from build123d import *

# Parameters (mm, degrees)
SKETCH_W        = 100
SKETCH_H        = 84
PAD_DEPTH       = 10
SKETCH001_R     = 2.1
POCKET_DEPTH    = 10
SKETCH002_R     = 3.2
POCKET001_DEPTH = 10
SKETCH003_R     = 4
POCKET002_DEPTH = 5
POCKET003_DEPTH = 4
SKETCH004_R     = 4.9
POCKET004_DEPTH = 5.2
FILLET_R        = 2
FILLET001_R     = 0.8
FILLET002_R     = 0.8


with BuildPart() as part:
    # Sketch → Pad (new body)
    with BuildSketch(Plane.XY):
        with Locations((50, 42)):
            Rectangle(SKETCH_W, SKETCH_H)
    extrude(amount=PAD_DEPTH)

    # Sketch001 (on Face6 of Pad) → Pocket (cut)
    with BuildSketch(Plane.XY.offset(10)):
        with Locations((6, 78)):
            Circle(SKETCH001_R)
        with Locations((30, 78)):
            Circle(SKETCH001_R)
        with Locations((6, 60)):
            Circle(SKETCH001_R)
        with Locations((30, 60)):
            Circle(SKETCH001_R)
        with Locations((6, 24)):
            Circle(SKETCH001_R)
        with Locations((30, 24)):
            Circle(SKETCH001_R)
        with Locations((6, 6)):
            Circle(SKETCH001_R)
        with Locations((30, 6)):
            Circle(SKETCH001_R)
        with Locations((70, 78)):
            Circle(SKETCH001_R)
        with Locations((94, 78)):
            Circle(SKETCH001_R)
        with Locations((70, 60)):
            Circle(SKETCH001_R)
        with Locations((94, 60)):
            Circle(SKETCH001_R)
        with Locations((70, 24)):
            Circle(SKETCH001_R)
        with Locations((94, 24)):
            Circle(SKETCH001_R)
        with Locations((70, 6)):
            Circle(SKETCH001_R)
        with Locations((94, 6)):
            Circle(SKETCH001_R)
        with Locations((35, 47)):
            Circle(SKETCH001_R)
        with Locations((65, 47)):
            Circle(SKETCH001_R)
        with Locations((35, 37)):
            Circle(SKETCH001_R)
        with Locations((65, 37)):
            Circle(SKETCH001_R)
    extrude(amount=-POCKET_DEPTH, mode=Mode.SUBTRACT)

    # Sketch002 (on Face5 of Pocket) → Pocket001 (cut)
    with BuildSketch(Plane.XY.offset(10)):
        with Locations((20, 62)):
            Circle(SKETCH002_R)
        with Locations((20, 22)):
            Circle(SKETCH002_R)
        with Locations((80, 62)):
            Circle(SKETCH002_R)
        with Locations((80, 22)):
            Circle(SKETCH002_R)
    extrude(amount=-POCKET001_DEPTH, mode=Mode.SUBTRACT)

    # Sketch003 (on Face5 of Pocket001) → Pocket002 (cut)
    with BuildSketch(Plane.XY.offset(10)):
        with Locations((6, 78)):
            Circle(SKETCH003_R)
        with Locations((30, 78)):
            Circle(SKETCH003_R)
        with Locations((30, 60)):
            Circle(SKETCH003_R)
        with Locations((6, 60)):
            Circle(SKETCH003_R)
        with Locations((70, 78)):
            Circle(SKETCH003_R)
        with Locations((94, 78)):
            Circle(SKETCH003_R)
        with Locations((70, 60)):
            Circle(SKETCH003_R)
        with Locations((94, 60)):
            Circle(SKETCH003_R)
        with Locations((6, 24)):
            Circle(SKETCH003_R)
        with Locations((30, 24)):
            Circle(SKETCH003_R)
        with Locations((6, 6)):
            Circle(SKETCH003_R)
        with Locations((30, 6)):
            Circle(SKETCH003_R)
        with Locations((70, 24)):
            Circle(SKETCH003_R)
        with Locations((94, 24)):
            Circle(SKETCH003_R)
        with Locations((70, 6)):
            Circle(SKETCH003_R)
        with Locations((94, 6)):
            Circle(SKETCH003_R)
        with Locations((35, 47)):
            Circle(SKETCH003_R)
        with Locations((35, 37)):
            Circle(SKETCH003_R)
        with Locations((65, 37)):
            Circle(SKETCH003_R)
        with Locations((65, 47)):
            Circle(SKETCH003_R)
    extrude(amount=-POCKET002_DEPTH, mode=Mode.SUBTRACT)

    # Sketch003 (on Face5 of Pocket001) → Pocket003 (cut)
    with BuildSketch(Plane.XY.offset(10)):
        with Locations((6, 78)):
            Circle(SKETCH003_R)
        with Locations((30, 78)):
            Circle(SKETCH003_R)
        with Locations((30, 60)):
            Circle(SKETCH003_R)
        with Locations((6, 60)):
            Circle(SKETCH003_R)
        with Locations((70, 78)):
            Circle(SKETCH003_R)
        with Locations((94, 78)):
            Circle(SKETCH003_R)
        with Locations((70, 60)):
            Circle(SKETCH003_R)
        with Locations((94, 60)):
            Circle(SKETCH003_R)
        with Locations((6, 24)):
            Circle(SKETCH003_R)
        with Locations((30, 24)):
            Circle(SKETCH003_R)
        with Locations((6, 6)):
            Circle(SKETCH003_R)
        with Locations((30, 6)):
            Circle(SKETCH003_R)
        with Locations((70, 24)):
            Circle(SKETCH003_R)
        with Locations((94, 24)):
            Circle(SKETCH003_R)
        with Locations((70, 6)):
            Circle(SKETCH003_R)
        with Locations((94, 6)):
            Circle(SKETCH003_R)
        with Locations((35, 47)):
            Circle(SKETCH003_R)
        with Locations((35, 37)):
            Circle(SKETCH003_R)
        with Locations((65, 37)):
            Circle(SKETCH003_R)
        with Locations((65, 47)):
            Circle(SKETCH003_R)
    extrude(amount=-POCKET003_DEPTH, mode=Mode.SUBTRACT)

    # Sketch004 (on Face4 of Pocket003) → Pocket004 (cut)
    with BuildSketch(Plane(origin=(0, 0, 0), x_dir=(1, 0, 0), z_dir=(0, 0, -1))):
        with Locations((20, -22)):
            Circle(SKETCH004_R)
        with Locations((80, -22)):
            Circle(SKETCH004_R)
        with Locations((20, -62)):
            Circle(SKETCH004_R)
        with Locations((80, -62)):
            Circle(SKETCH004_R)
    extrude(amount=-POCKET004_DEPTH, mode=Mode.SUBTRACT)

    # Fillet
    fillet_edges = [part.edges().sort_by_distance(p)[0] for p in [
        (100, 0, 5),
        (100, 84, 5),
        (0, 84, 5),
        (0, 0, 5),
    ]]
    fillet(fillet_edges, radius=FILLET_R)

    # Fillet001
    fillet001_edges = [part.edges().sort_by_distance(p)[0] for p in [
        (100, 42, 10),
        (99.414214, 0.585786, 10),
        (50, 0, 10),
        (0.585786, 0.585786, 10),
        (0, 42, 10),
        (0.585786, 83.414214, 10),
        (50, 84, 10),
        (99.414214, 83.414214, 10),
    ]]
    fillet(fillet001_edges, radius=FILLET001_R)

    # Fillet002
    fillet002_edges = [part.edges().sort_by_distance(p)[0] for p in [
        (0, 42, 0),
        (0.585786, 0.585786, 0),
        (50, 0, 0),
        (99.414214, 0.585786, 0),
        (100, 42, 0),
        (99.414214, 83.414214, 0),
        (50, 84, 0),
        (0.585786, 83.414214, 0),
    ]]
    fillet(fillet002_edges, radius=FILLET002_R)


solid = part.part
For this review, take the finished solid that the model builds, in its own axes (mm). A direction names the side the tool comes from. Coordinates: 2 decimals unless noted, no trailing zeros. Order: outer loops, then holes, each group sorted by start corner. A loop starts at its lowest first (then second) coordinate and runs counter-clockwise, first axis right, second up. Notation, with made-up numbers: (42, -37) - (87, -37) arc R9 ccw to (87, -33) - close; hole circle Ø8 at (78, 88). An arc over 180 degrees is marked (long way). Answer as CSV lines item,"result". Start each with the question number.
1) Add section C-C (z = 2). Count the separate pieces of the cut face and the enclosed holes in it, then the cut area to 3 significant figures.
2) Machinability: for faces 4 (the cylindrical face through (91.9, 6.09, 2.54)), 5 (the flat face through (23.2, 23, 5.2)), 6 (the flat face through (72, 22, 5)), which of the approach directions +Z, -Z, +X, -X, +Y, -Y give a long, thin tool a straight path to every point of the face, cutting with its end or side? Answer none if there is none.
3) Add section B-B (y = 37). State the section outline as (x, z) points, then the cut area to 3 significant figures.
4) Add section A-A (x = 80). State the section outline as (y, z) points.
5) Draft analysis for pull direction Y (two halves, no side actions). For faces 1 (the flat face through (0, 41, 5)), 2 (the cylindrical face through (0.57, 83.4, 5.06)), 3 (the cylindrical face through (33.334, 35.722, 2.535)), state which applies: +Y half, -Y half, draft (parallel to the pull), parting line (faces both ways), or undercut.
6) Insertion check: P1, Ø4, axis at x = 70, y = 6, coming from the +Z side; P2, Ø6.5, axis at x = 30, y = 24, coming from the +Z side. Each pin has a flat end and moves straight along its axis. Give the tip position at first contact, or say it passes through.
7) To check wall thickness, follow line 1 along Y through (x, z) = (65, 6.6); line 2 along Y through (x, z) = (94, 2.95); line 3 along X through (y, z) = (58, 9.25). State the ranges of each line that lie inside material, in increasing order. Write a range as [from, to].
Result:
1,separate pieces,"1"
1,enclosed holes,"24"
1,area,"7,820 mm^2"
2,face 4,"+Z, -Z"
2,face 5,"-Z"
2,face 6,"+Z"
3,outline,"(0, 0.8) arc R0.8 ccw to (0.8, 0) - (32.9, 0) - (32.9, 5) - (31, 5) - (31, 10) - (0.8, 10) arc R0.8 ccw to (0, 9.2) - close; (37.1, 0) - (62.9, 0) - (62.9, 5) - (61, 5) - (61, 10) - (39, 10) - (39, 5) - (37.1, 5) - close; (67.1, 0) - (99.2, 0) arc R0.8 ccw to (100, 0.8) - (100, 9.2) arc R0.8 ccw to (99.2, 10) - (69, 10) - (69, 5) - (67.1, 5) - close"
3,area,"877 mm^2"
4,outline,"(0, 0.8) arc R0.8 ccw to (0.8, 0) - (17.1, 0) - (17.1, 5.2) - (18.8, 5.2) - (18.8, 10) - (0.8, 10) arc R0.8 ccw to (0, 9.2) - close; (25.2, 5.2) - (26.9, 5.2) - (26.9, 0) - (57.1, 0) - (57.1, 5.2) - (58.8, 5.2) - (58.8, 10) - (25.2, 10) - close; (65.2, 5.2) - (66.9, 5.2) - (66.9, 0) - (83.2, 0) arc R0.8 ccw to (84, 0.8) - (84, 9.2) arc R0.8 ccw to (83.2, 10) - (65.2, 10) - close"
5,face 1,"draft"
5,face 2,"+Y half"
5,face 3,"undercut"
6,P1,"through"
6,P2,"z = 5"
7,line 1,"[0, 33], [41, 43], [51, 84]"
7,line 2,"[0, 3.9], [8.1, 21.9], [26.1, 57.9], [62.1, 75.9], [80.1, 84]"
7,line 3,"[0, 2.54], [9.46, 26.54], [33.46, 66.54], [73.46, 90.54], [97.46, 100]"
